Input: part model. Units: mm. Frame: model coordinates. A direction names the side the tool comes from. Coordinates: 2 decimals unless noted, no trailing zeros. Write each loop counter-clockwise with the first axis right and the second up, starting at its lowest first coordinate (ties: lowest second). Pieces come first, ordered by that corner, then holes. Notation, with made-up numbers: (4, -17) -> (35, -17) arc R15 ccw to (35, 11) -> close; hole circle Ø4 at (3, 39). An arc over 180 degrees is marked (long way). Use one line per item in the form item = value. Start each with the question number.
(1) Pull-direction query (Z, two-part tool) for faces 1 (the face through (0, -45, 15)), 2 (the face through (41, 1, 0)), 3 (the face through (41, 1, 30)); classes: released by +Z, released by -Z, zero draft, split by the parting line, or undercut.
(2) Cut plane C-C on x = 42.5. Return the cut outline in (y, z).
(3) Cut plane A-A on x = 5. Return the cut outline in (y, z).
(4) Cut plane D-D on y = -32. Return the cut outline in (x, z).
(5) Ray query, line 1 along Y through (x, z) = (22, 14.5); line 2 along Y through (x, z) = (15.5, 17.5); line 3 along Y through (x, z) = (42, 15). Return the intervals inside material, ascending.
(6) Cut plane B-B on z = 21.75. Return the cut outline in (x, y).
(7) Set-up query: faces 4 (the face through (50, -1, 15)), 5 (the face through (40, 37, 15)), 6 (the face through (31, -43, 15)). Return all of +Z, -Z, +X, -X, +Y, -Y with unobstructed straight access to the full face (end or side cutting, diameter ignored); none if empty.
```python
from build123d import *

# Parameters (mm, degrees)
EXTRUDE_1_DEPTH     = 30
SKETCH_2_W          = 19
SKETCH_2_H          = 13
CUT_EXTRUDE_1_DEPTH = 77.811457479


with BuildPart() as part:
    # Эскиз1 → Бобышка-Вытянуть1 (new body)
    with BuildSketch(Plane.XY):
        with BuildLine():
            Line((50, 50), (0, 50))
            Line((0, 50), (0, 40))
            ThreePointArc((0, 40), (28.284271247, 28.284271247), (40, 0))
            ThreePointArc((40, 0), (28.284271247, -28.284271247), (0, -40))
            Line((0, -40), (0, -50))
            Line((0, -50), (50, -50))
            Line((50, -50), (50, 50))
        make_face()
    extrude(amount=EXTRUDE_1_DEPTH)

    # Эскиз2 → Вырез-Вытянуть1 (cut, through all)
    with BuildSketch(Plane.XY.offset(30)):
        with Locations((40.5, 43.5)):
            Rectangle(SKETCH_2_W, SKETCH_2_H)
    cut_extrude_1 = extrude(amount=-CUT_EXTRUDE_1_DEPTH, mode=Mode.SUBTRACT)

    # Зеркальное отражение1: Вырез-Вытянуть1 across plane
    add(cut_extrude_1.mirror(Plane.ZX), mode=Mode.SUBTRACT)


solid = part.part
```
Values:
q1.face_1 = zero draft
q1.face_2 = released by -Z
q1.face_3 = released by +Z
q2.outline = (-37, 0) -> (37, 0) -> (37, 30) -> (-37, 30) -> close
q3.outline = (-50, 0) -> (-39.69, 0) -> (-39.69, 30) -> (-50, 30) -> close; (39.69, 0) -> (50, 0) -> (50, 30) -> (39.69, 30) -> close
q4.outline = (24, 0) -> (50, 0) -> (50, 30) -> (24, 30) -> close
q5.line_1 = -50 to -33.41, 33.41 to 50
q5.line_2 = -50 to -36.87, 36.87 to 50
q5.line_3 = -37 to 37
q6.outline = (0, -50) -> (31, -50) -> (31, -37) -> (50, -37) -> (50, 37) -> (31, 37) -> (31, 50) -> (0, 50) -> (0, 40) arc R40 cw to (0, -40) -> close
q7.face_4 = +Z, -Z, +X, +Y, -Y
q7.face_5 = +Z, -Z, +X, +Y
q7.face_6 = +Z, -Z, +X, -Y
